For this review, take the finished solid that the model builds, in its own axes (mm). Face numbers are marked on the shaded views. A direction names the side the tool comes from. Coordinates: 2 decimals unless noted, no trailing zeros. Order: outer loops, then holes, each group sorted by start corner. A loop starts at its lowest first (then second) coordinate and runs counter-clockwise, first axis right, second up. Notation, with made-up numbers: M -8,79 L 24,79 A25 cw 24,91 Z; hole C 48,27.25 d3. An arc over 180 degrees is marked long. Use CSV: the item, a comma, the result in double quotes.
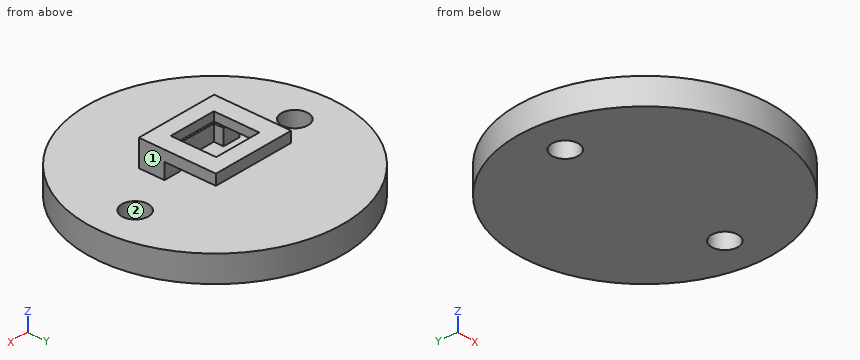
```python
from build123d import *

# Parameters (mm, degrees)
F0_R     = 14.460691
F0_R_2   = 1.5
F1_DEPTH = 3
F2_W     = 9.428674
F2_H     = 8.726458
F2_W_2   = 5.4
F2_H_2   = 5.150138
F3_DEPTH = 3
F4_W     = 15.93314
F4_H     = 7.691861
F5_DEPTH = 1.8
F6_W     = 6.640965
F6_H     = 6.223533
F7_DEPTH = 0.2


with BuildPart() as f1:
    # F0 (on Top) → F1 (new body)
    with BuildSketch(Plane.XY):
        Circle(F0_R)
        with Locations((-10, 0)):
            Circle(F0_R_2, mode=Mode.SUBTRACT)
        with Locations((10, 0)):
            Circle(F0_R_2, mode=Mode.SUBTRACT)
    extrude(amount=F1_DEPTH)

    # F2 (on face) → F3 (join)
    with BuildSketch(Plane.XY.offset(3)):
        Rectangle(F2_W, F2_H)
        Rectangle(F2_W_2, F2_H_2, mode=Mode.SUBTRACT)
    extrude(amount=F3_DEPTH)

    # F4 (on face) → F5 (cut)
    with BuildSketch(Plane.XY.offset(3)):
        with Locations((-0.366279, 2.380814)):
            Rectangle(F4_W, F4_H)
    extrude(amount=F5_DEPTH, mode=Mode.SUBTRACT)

    # F6 (on face) → F7 (cut)
    with BuildSketch(Plane(origin=(0, 0, 4.8), x_dir=(1, 0, 0), z_dir=(0, 0, -1))):
        with Locations((-0.009842, 0.080773)):
            Rectangle(F6_W, F6_H)
    extrude(amount=-F7_DEPTH, mode=Mode.SUBTRACT)


solid = f1.part
```
Item 1: Add section C-C on z = 5.5. State the section outline as (x, y) points.
Solutions:
outline,"M -4.71,-4.36 L 4.71,-4.36 L 4.71,4.36 L -4.71,4.36 Z; hole M -2.7,-2.58 L 2.7,-2.58 L 2.7,2.58 L -2.7,2.58 Z"
Item 2: Clearance check with flat-ended pins moving along their axes: pin 1 Ø0.5 at (y, z) = (-0.5, 5.5) entering from -X; pin 2 Ø6 at (x, y) = (-9.5, -9) entering from +Z; pin 3 Ø4.5 at (x, y) = (-0.5, 2.5) entering from -Z; pin 4 Ø1 at (y, z) = (8, 1) entering from -X. State where each tip first meets the part, or that it passes through.
Solutions:
pin 1,"x = -4.71"
pin 2,"z = 3"
pin 3,"z = 0"
pin 4,"x = -12.36"
Item 3: Add section D-D on z = 4.05. State the section outline as (x, y) points, and give its area (3 significant figures).
Solutions:
outline,"M -4.71,-4.36 L 4.71,-4.36 L 4.71,-1.47 L 2.7,-1.47 L 2.7,-2.58 L -2.7,-2.58 L -2.7,-1.47 L -4.71,-1.47 Z"
area,"21.3 mm^2"
Item 4: To check wall thickness, follow line 1 along Z through (x, y) = (3.5, 4); line 2 along X through (y, z) = (-2.25, 4.05); line 3 along Y through (x, z) = (9.5, 2.4). State the ranges of each line that lie inside material, in increasing order. Write a range as [from, to].
Solutions:
line 1,"[0, 3], [4.8, 6]"
line 2,"[-4.71, -2.7], [2.7, 4.71]"
line 3,"[-10.9, -1.41], [1.41, 10.9]"
Item 5: Add section A-A on y = 0. State the section outline as (x, z) points.
Solutions:
outline,"M -14.46,0 L -11.5,0 L -11.5,3 L -14.46,3 Z; M -8.5,0 L 8.5,0 L 8.5,3 L -8.5,3 Z; M -4.71,4.8 L -3.33,4.8 L -3.33,5 L -2.7,5 L -2.7,6 L -4.71,6 Z; M 2.7,5 L 3.31,5 L 3.31,4.8 L 4.71,4.8 L 4.71,6 L 2.7,6 Z; M 11.5,0 L 14.46,0 L 14.46,3 L 11.5,3 Z"
Item 6: Add section B-B on x = 0. State the section outline as (y, z) points.
Solutions:
outline,"M -14.46,0 L 14.46,0 L 14.46,3 L -2.58,3 L -2.58,4.8 L -3.19,4.8 L -3.19,5 L -2.58,5 L -2.58,6 L -4.36,6 L -4.36,3 L -14.46,3 Z; M 2.58,5 L 3.03,5 L 3.03,4.8 L 4.36,4.8 L 4.36,6 L 2.58,6 Z"
Item 7: For the marked faces 1 and 2, list the 3-axis set-ups (+Z, -Z, +X, -X, +Y, -Y) from which the entire face can be reached by the end or side of a thin tool; tool diameter is ignored.
Solutions:
face 1,"+Z, +X, +Y, -Y"
face 2,"+Z, -Z"
